Here's the drawing with two shaded views (mm, measured from the low corner). I have some questions. A direction names the side the tool comes from. Coordinates: 2 decimals unless noted, no trailing zeros. Write each loop counter-clockwise with the first axis right and the second up, starting at its lowest first coordinate (ties: lowest second). Pieces come first, ordered by that corner, then holes.
Item 1: If I drill on probe 1 along X at (y, z) = (19, 4); probe 2 along Y at (x, z) = (20.5, 3.5), over which ranges is the centre line in solid material (lowest first)?
Item 2: Which directions (+Z, -Z, +X, -X, +Y, -Y) give clear straight access to the entire face, cutting with the end or side of a thin tool? Please do the marked faces 1 and 2.
Item 3: I want a section at B-B on x = 25. Please give me the cut outline in (y, z).
Item 4: I want a section at A-A on y = 13.5. Please give me the cut outline in (x, z), then the cut area to 3 significant figures.
Item 5: I want a section at C-C on z = 9.25. Please give me the cut outline in (x, y), then the cut area to 3 significant figures.
Item 6: For P1, Ø2, axis at y = 10.5, z = 5.5, coming from the +X side; P2, Ø9.5, axis at x = 25.5, z = 12.5, coming from the -Y side, each with a flat end and sliding along its axis, tell me the tip position at first contact or that it passes through.
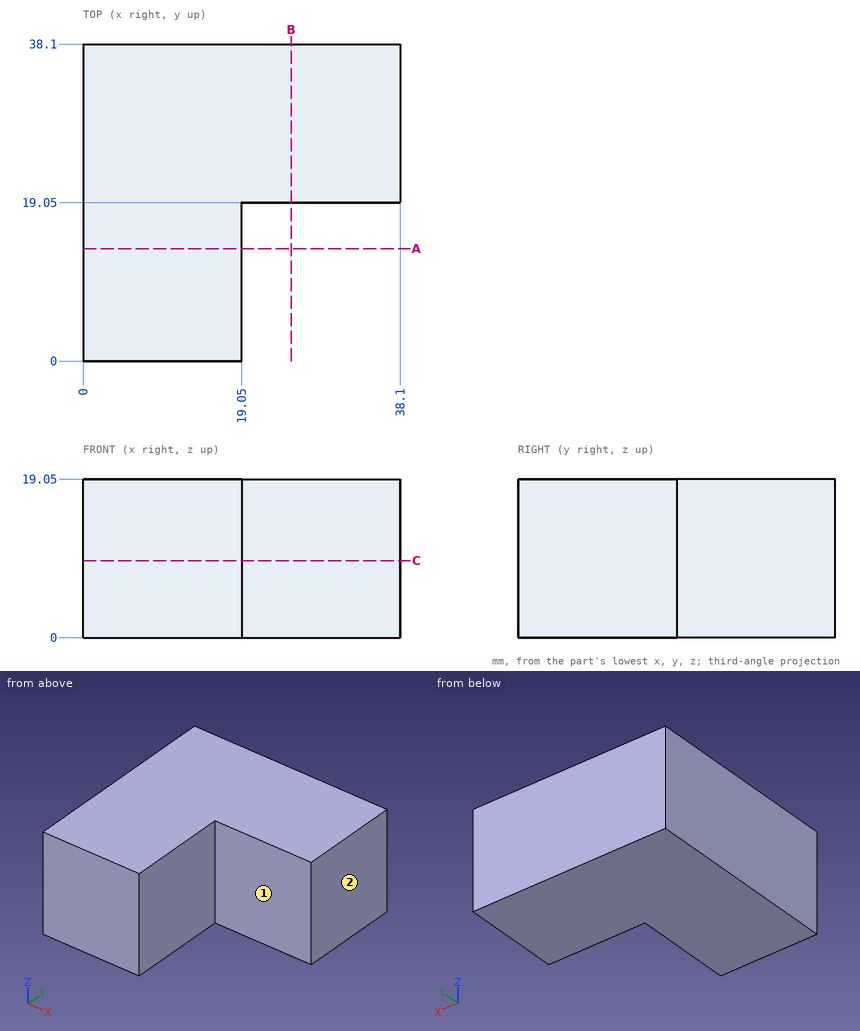
Response values:
1. probe 1: x = 0 to 19.05
1. probe 2: y = 19.05 to 38.1
2. face 1: +Z, -Z, +X, -Y
2. face 2: +Z, -Z, +X, +Y, -Y
3. outline: (19.05, 0) - (38.1, 0) - (38.1, 19.05) - (19.05, 19.05) - close
4. outline: (0, 0) - (19.05, 0) - (19.05, 19.05) - (0, 19.05) - close
4. area: 363 mm2
5. outline: (0, 0) - (19.05, 0) - (19.05, 19.05) - (38.1, 19.05) - (38.1, 38.1) - (0, 38.1) - close
5. area: 1,090 mm2
6. P1: stops at x = 19.05
6. P2: stops at y = 19.05
